Check sheet for the drawn part. Datum: minimum x, y, z corner. Units: mm. A direction names the side the tool comes from. Coordinates: 2 decimals unless noted, no trailing zeros. Write each loop counter-clockwise with the first axis right and the second up, starting at its lowest first coordinate (ties: lowest second). Pieces come first, ordered by that corner, then holes. Notation, with made-up numbers: (69.25, -16) -> (76.25, -16) arc R13 cw to (76.25, -4) -> close; hole circle Ø7 at (60, -39). An arc over 180 degrees is marked (long way). One line per question, with ' | ' between items.
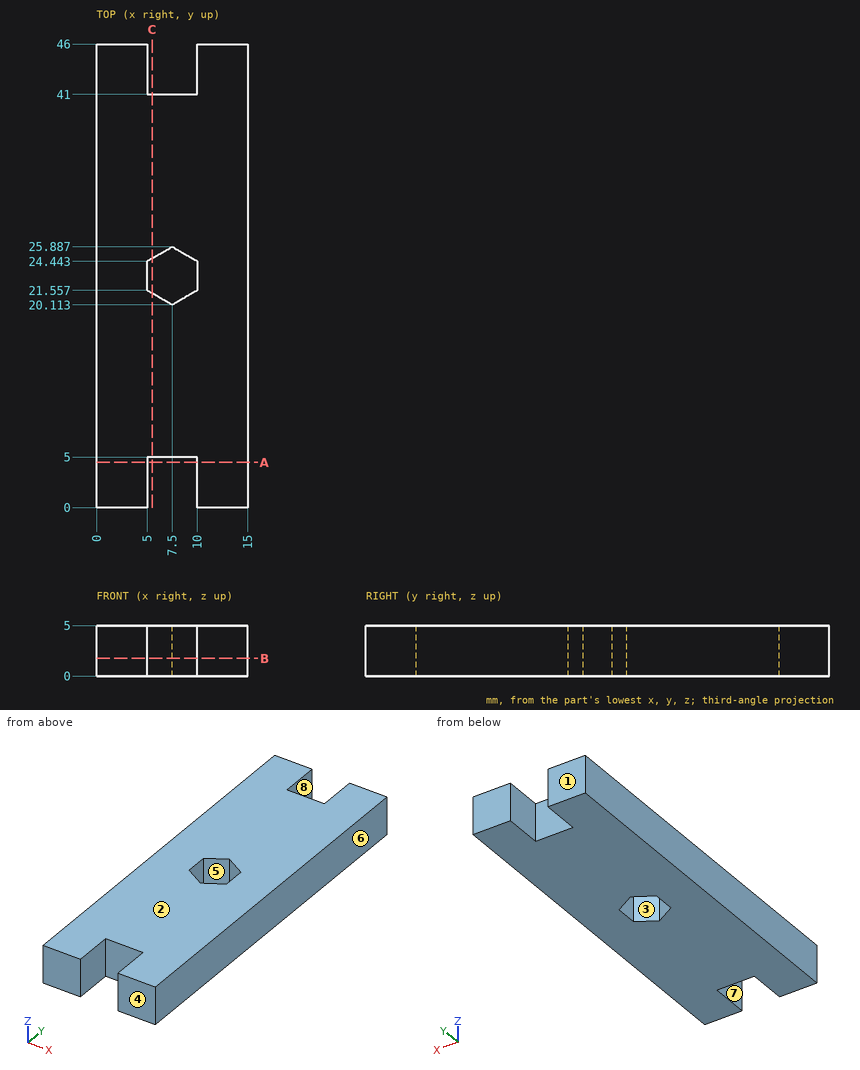
1. Tool access check on the marked faces 4, 5, 6, 7 and 8. Record the directions out of +Z, -Z, +X, -X, +Y, -Y that give a thin tool (end or side, any length) a straight path to the whole face; none if there is none.
Worked answers:
face 4: +Z, -Z, +X, -X, -Y | face 5: +Z, -Z | face 6: +Z, -Z, +X, +Y, -Y | face 7: +Z, -Z, -Y | face 8: +Z, -Z, +Y
2. Cross-section at C-C on x = 5.5. Record the boundary of the cut face in (y, z), and give its area (3 significant figures).
Worked answers:
outline: (5, 0) -> (21.27, 0) -> (21.27, 5) -> (5, 5) -> close; (24.73, 0) -> (41, 0) -> (41, 5) -> (24.73, 5) -> close | area: 163 mm²
3. Mould release check, pull along Y, two halves, no side actions. Record for the marked faces 1, 2 and 3: released by +Y, released by -Y, zero draft, split by the parting line, or undercut.
Worked answers:
face 1: released by +Y | face 2: zero draft | face 3: undercut
4. Material ranges on line 1 (Y direction, x = 7.5, z = 3.6); line 2 (X direction, y = 3.5, z = 0.4); line 3 (Y direction, x = 8.75, z = 2.1) (1 decimal), recorded low to high. Write a range as from..to.
Worked answers:
line 1: 5..20.11, 25.89..41 | line 2: 0..5, 10..15 | line 3: 5..20.8, 25.2..41
5. Cross-section at A-A on y = 4.5. Record the boundary of the cut face in (x, z), and give its area (3 significant figures).
Worked answers:
outline: (0, 0) -> (5, 0) -> (5, 5) -> (0, 5) -> close; (10, 0) -> (15, 0) -> (15, 5) -> (10, 5) -> close | area: 50.0 mm²
6. Cross-section at B-B on z = 1.75. Record the boundary of the cut face in (x, y).
Worked answers:
outline: (0, 0) -> (5, 0) -> (5, 5) -> (10, 5) -> (10, 0) -> (15, 0) -> (15, 46) -> (10, 46) -> (10, 41) -> (5, 41) -> (5, 46) -> (0, 46) -> close; hole (5, 21.56) -> (7.5, 20.11) -> (10, 21.56) -> (10, 24.44) -> (7.5, 25.89) -> (5, 24.44) -> close
7. Go/stop test with a flat-tipped pin: P1, Ø1, axis at x = 7, z = 1.5, coming from the +Y side. Record where the tip stops, or that it passes through.
Worked answers:
P1: y = 41
